```python
from build123d import *

# Parameters (mm, degrees)
RESSALTO_EXTRUS_O4_DEPTH = 5
ESBO_O8_R                = 1.8
CORTE_EXTRUS_O3_DEPTH    = 112.673524207
RESSALTO_EXTRUS_O5_START = -8
RESSALTO_EXTRUS_O5_DEPTH = 8
CORTE_EXTRUS_O4_DEPTH    = 3
FILETE1_R                = 5
FILETE2_R                = 2


with BuildPart() as part:
    # Esboço6 → Ressalto-extrusão4 (new body)
    with BuildSketch(Plane(origin=(0, 0, 0), x_dir=(1, 0, 0), z_dir=(0, 1, 0))):
        with BuildLine():
            Line((0, -82.26), (0, -108.5))
            ThreePointArc((0, -108.5), (-13.073364664, -107.709503464), (-25.956232563, -105.349532468))
            Line((-25.956232563, -105.349532468), (-14.581921132, -80.957242888))
            ThreePointArc((-14.581921132, -80.957242888), (-7.32, -81.933663411), (0, -82.26))
        make_face()
    extrude(amount=RESSALTO_EXTRUS_O4_DEPTH)

    # Esboço8 → Corte-extrusão3 (cut, through all)
    with BuildSketch(Plane(origin=(0, 5, 0), x_dir=(1, 0, 0), z_dir=(0, 1, 0))):
        with Locations(Location((-5, -95.38, 0), (0, 0, 270))):
            Circle(ESBO_O8_R)
    extrude(amount=-CORTE_EXTRUS_O3_DEPTH, mode=Mode.SUBTRACT)

    # Esboço7 → Ressalto-extrusão5 (add)
    with BuildSketch(Plane(origin=(0, 5, 0), x_dir=(1, 0, 0), z_dir=(0, 1, 0)).offset(RESSALTO_EXTRUS_O5_START)):
        with BuildLine():
            ThreePointArc((0, -108.5), (1.893586098, -108.483474924), (3.786595392, -108.433904732))
            Line((3.786595392, -108.433904732), (2.870832599, -82.209889431))
            ThreePointArc((2.870832599, -82.209889431), (1.435634954, -82.247471404), (0, -82.26))
            Line((0, -82.26), (0, -108.5))
        make_face()
    extrude(amount=RESSALTO_EXTRUS_O5_DEPTH)

    # Esboço9 → Corte-extrusão4 (cut)
    with BuildSketch(Plane(origin=(0, 5, 0), x_dir=(1, 0, 0), z_dir=(0, 1, 0))):
        Polygon((-7.75, -93.79228676), (-7.75, -96.96771324), (-5, -98.555426481), (-2.25, -96.96771324), (-2.25, -93.79228676), (-5, -92.204573519), align=None)
    extrude(amount=-CORTE_EXTRUS_O4_DEPTH, mode=Mode.SUBTRACT)

    # Filete1
    filete1_edges = [part.edges().sort_by_distance(p)[0] for p in [
        (-14.581921132, 2.5, 80.957242888),
    ]]
    fillet(filete1_edges, radius=FILETE1_R)

    # Filete2
    # the kernel refuses this fillet: 2 mm, written as the material it takes off along each edge
    with BuildSketch(Plane(origin=(-25.956232563, -6.211327666, 105.349532468), x_dir=(0.42261826174069944, 0, -0.9063077870366499), z_dir=(0, 1, 0))) as filete2_piece_1:
        with BuildLine():
            CenterArc((2.461525654, -2), FILETE2_R, 90, 102.471061381)
            ThreePointArc((0.508715252, -2.431892969), (0.247396438, -1.21740266), (0, 0))
            Line((0, 0), (2.461525654, 0))
        make_face()
    extrude(amount=17.422655332, mode=Mode.SUBTRACT)
    with BuildSketch(Plane(origin=(2.870832599, -7.940651502, 82.209889431), x_dir=(-0.9997346498502194, 0, 0.023035405116018468), z_dir=(0, 1, 0))) as filete2_piece_2:
        with BuildLine():
            CenterArc((1.976403158, 1.999859125), FILETE2_R, 180.680051756, 88.639896488)
            Line((-0.023455967, 1.976121398), (0, 0))
            ThreePointArc((0, 0), (0.976332715, 0.005794184), (1.952665431, 0))
        make_face()
    extrude(amount=17.881303004, mode=Mode.SUBTRACT)
    with BuildSketch(Plane(origin=(3.786595392, -8.094121302, 108.433904732), x_dir=(-0.034899496702502156, 0, -0.9993908270190958), z_dir=(0, 1, 0))) as filete2_piece_3:
        with BuildLine():
            CenterArc((2.018780999, 2), FILETE2_R, 178.923959667, 91.076040333)
            ThreePointArc((0.019133694, 2.037558685), (0.004783529, 1.01882426), (0, 0))
            Line((0, 0), (2.018780999, 0))
        make_face()
    extrude(amount=18.188242605, mode=Mode.SUBTRACT)
    with BuildSketch(Plane(origin=(0, -7.940651502, 82.26), x_dir=(0.9999295625583442, 0, -0.011868863546203106), z_dir=(0, 1, 0))) as filete2_piece_4:
        with BuildLine():
            CenterArc((1.976403158, -1.999859125), FILETE2_R, 90.680051756, 88.639896488)
            Line((-0.023455967, -1.976121398), (0, 0))
            ThreePointArc((0, 0), (0.976332715, -0.005794184), (1.952665431, 0))
        make_face()
    extrude(amount=7.940651502, mode=Mode.SUBTRACT)


solid = part.part
```
The model under review builds one solid part; all positions refer to its coordinate system, in mm. A direction names the side the tool comes from. Round coordinates to 2 decimals unless told otherwise and drop trailing zeros. Order: outer loops, then holes, each group sorted by start corner. A loop starts at its lowest first (then second) coordinate and runs counter-clockwise, first axis right, second up. Notation, with made-up numbers: M 9.5,13.25 L 32.5,13.25 A4 ccw 32.5,17.25 Z; hole C -13,68.25 d6. An arc over 180 degrees is marked long. Use a Markdown table: item, result.
1) Consider section C-C (y = 3). Write out the cut boundary in (x, z), then the cut area to 3 significant figures.
Report:
| item | result |
|---|---|
| outline | M -24.92,103.12 L -16.17,84.37 A5 ccw -10.97,81.52 A82.26 cw 0,82.26 A82.26 cw 0.92,82.25 A2 ccw 2.94,84.18 L 3.72,106.42 A2 ccw 1.75,108.49 A108.5 ccw 0,108.5 A108.5 ccw -23.54,105.92 A2 ccw Z; hole M -7.75,93.79 L -5,92.2 L -2.25,93.79 L -2.25,96.97 L -5,98.56 L -7.75,96.97 Z |
| area | 592 mm^2 |
2) Insertion check: pin 1 (1.5 mm diameter, centred on x = -15.5, y = 2.5, fed in from -Z); pin 2 (13.5 mm diameter, centred on x = -9, z = 96.5, fed in from -Y); pin 3 (1 mm diameter, centred on y = 1, z = 89, fed in from +X); pin 4 (4 mm diameter, centred on x = -13, y = 0, fed in from -Z). Each pin has a flat end and moves straight along its axis. Give the tip position at first contact, or say it passes through.
Report:
| item | result |
|---|---|
| pin 1 | z = 82.56 |
| pin 2 | y = 0 |
| pin 3 | x = 3.13 |
| pin 4 | z = 81.48 |
3) Wall thickness on line 1 along Y through (x, z) = (-2.25, 90.5); line 2 along Z through (x, y) = (-4.5, 3.25); line 3 along Z through (x, y) = (1, 1.75): over which ranges is each line inside the solid? List them lowest first. Write a range as [from, to].
Report:
| item | result |
|---|---|
| line 1 | [0, 5] |
| line 2 | [82.14, 92.49], [98.27, 108.41] |
| line 3 | [82.26, 108.5] |
4) Consider section D-D (z = 87.5). Write out the cut boundary in (x, y), then the cut area to 3 significant figures.
Report:
| item | result |
|---|---|
| outline | M -17.63,0 L 0,0 L 0,-3 L 3.06,-3 L 3.06,5 L -17.63,5 Z |
| area | 113 mm^2 |
5) Draft analysis for pull direction X (two halves, no side actions). For faces 1 (the face through (-24.908, 2.465, 104.825)), 2 (the face through (-12, 0, 95)), 3 (the face through (3.15, 0.94, 107.88)), 4 (the face through (-7.75, 4, 95)), state which applies: released by +X, released by -X, zero draft, split by the parting line, or undercut.
Report:
| item | result |
|---|---|
| face 1 | released by -X |
| face 2 | zero draft |
| face 3 | released by +X |
| face 4 | undercut |
6) Consider section A-A (y = 1). Write out the cut boundary in (x, z).
Report:
| item | result |
|---|---|
| outline | M -24.92,103.12 L -16.17,84.37 A5 ccw -10.97,81.52 A82.26 cw 0,82.26 A82.26 cw 0.92,82.25 A2 ccw 2.94,84.18 L 3.72,106.42 A2 ccw 1.75,108.49 A108.5 ccw 0,108.5 A108.5 ccw -23.54,105.92 A2 ccw Z; hole C -5,95.38 d3.6 |
7) Tool access review of faces 5 (the face through (-6.394, 3.521, 97.75)), 6 (the face through (2, -3, 95)), 7 (the face through (0.41, -1.52, 83.02)): name each direction out of +Z, -Z, +X, -X, +Y, -Y from which nothing blocks a thin tool from reaching the whole face with its end or side.
Report:
| item | result |
|---|---|
| face 5 | +Y |
| face 6 | +Z, -Z, +X, -X, -Y |
| face 7 | -Z, -X, -Y |
8) Consider section B-B (z = 95). Write out the cut boundary in (x, y).
Report:
| item | result |
|---|---|
| outline | M -21.13,0 L -6.76,0 L -6.76,2 L -7.75,2 L -7.75,5 L -21.13,5 Z; M -3.24,0 L 0,0 L 0,-3 L 3.32,-3 L 3.32,5 L -2.25,5 L -2.25,2 L -3.24,2 Z |
